Geometry check sheet. Reference: the model listing, model coordinates, mm. A direction names the side the tool comes from. Give positions to 0.01 mm unless a question says otherwise; leave off trailing zeros. Loops run counter-clockwise (first coordinate to the right, second up) from the corner with the lowest first, then second, coordinate; pieces in that order, holes last. Notation, with made-up numbers: (79.25, 63.5) - (93.25, 63.5) arc R5 ccw to (93.25, 71.5) - close; hole circle Ø8 at (48, -5). An arc over 180 degrees is marked (long way). Use a Markdown table: item, result. Add a question column.
1. Set-up check for faces 5 (the cylindrical face through (-8.43, 8.36, 4.38)), 6 (the cylindrical face through (-16.856, -6.447, 8.767)), 7 (the flat face through (8, 20, 15)): record each of +Z, -Z, +X, -X, +Y, -Y from which the full face is reachable in a straight line by a thin tool's end or side.
2. Draft check along Y on faces 1 (the flat face through (0, 18.5, 21)), 2 (the flat face through (-4, -1.5, 9)), 3 (the flat face through (-1.4, 18.5, -8.1)), 4 (the cylindrical face through (0, 20, -8)). Enter one of: pulls with the +Y half, pulls with the -Y half, needs draft (parallel to the pull), parting line crosses it, or undercut.
3. Cross-section at B-B on y = 8. Enter the section's corners in (x, z), and give its area (3 significant figures).
4. Depth check by flat-ended pin: P1, Ø0.9, axis at y = 20, z = 14, coming from the -X side; P2, Ø2, axis at x = -11.5, y = -4.5, coming from the +Z side; P3, Ø1.5, axis at x = -4.5, y = -8.5, coming from the +Z side. Enter the tip coordinate at first touch or a pass-through.
5. Cross-section at C-C on z = 25. Enter the section's corners in (x, y).
6. Cross-section at A-A on x = 0. Enter the section's corners in (y, z), and give its area (3 significant figures).
7. Cross-section at D-D on y = -14. Enter the section's corners in (x, z), and give its area (3 significant figures).
8. Material ranges on L1, parallel to Y at x = 0, z = 20.5; L2, parallel to X at y = 7, z = -6; L3, parallel to Z at x = 3, y = 3.5, recorded low to high.
from build123d import *

# Parameters (mm, degrees)
F3_DEPTH = 3


with BuildPart() as f1:
    # F0 (on Right) → F1 (revolve)
    with BuildSketch(Plane.YZ):
        Polygon((-18.5, 9.559073), (-18.5, 0), (18.5, 0), (18.5, 9.5), (-1.5, 9.5), (-1.5, 19), (-11.25722, 19), align=None)
    revolve(axis=Axis((0, -2.898404, 0), (0, 1, 0)))

    # F2 (on face) → F3 (join)
    with BuildSketch(Plane(origin=(0, 18.5, 0), x_dir=(-1, 0, 0), z_dir=(0, 1, 0))):
        with BuildLine():
            ThreePointArc((8, 29), (0, 37), (-8, 29))
            Line((-8, 29), (-8, 5.123475))
            ThreePointArc((-8, 5.123475), (0, 9.5), (8, 5.123475))
            Line((8, 5.123475), (8, 29))
        make_face()
        with BuildLine():
            ThreePointArc((8, 5.123475), (0, 9.5), (-8, 5.123475))
            Line((-8, 5.123475), (-8, 0))
            ThreePointArc((-8, 0), (0, -8), (8, 0))
            Line((8, 0), (8, 5.123475))
        make_face()
    extrude(amount=F3_DEPTH)


solid = f1.part
Values found:
| question | item | result |
|---|---|---|
| 1 | face 5 | none |
| 1 | face 6 | -Y |
| 1 | face 7 | +Z, -Z, +X, +Y |
| 2 | face 1 | undercut |
| 2 | face 2 | undercut |
| 2 | face 3 | pulls with the +Y half |
| 2 | face 4 | needs draft |
| 3 | outline | circle Ø19 at (0, 0) |
| 3 | area | 284 mm2 |
| 4 | P1 | stops at x = -8 |
| 4 | P2 | stops at z = 15.84 |
| 4 | P3 | stops at z = 18.63 |
| 5 | outline | (-8, 18.5) - (8, 18.5) - (8, 21.5) - (-8, 21.5) - close |
| 6 | outline | (-18.5, -9.56) - (-11.26, -19) - (-1.5, -19) - (-1.5, -9.5) - (18.5, -9.5) - (18.5, -8) - (21.5, -8) - (21.5, 37) - (18.5, 37) - (18.5, 9.5) - (-1.5, 9.5) - (-1.5, 19) - (-11.26, 19) - (-18.5, 9.56) - close |
| 6 | area | 1,090 mm2 |
| 7 | outline | circle Ø30.85 at (0, 0) |
| 7 | area | 747 mm2 |
| 8 | L1 | y = 18.5 to 21.5 |
| 8 | L2 | x = -7.37 to 7.37 |
| 8 | L3 | z = -9.01 to 9.01 |
